```python
from build123d import *

# Parameters (mm, degrees)
F1_DEPTH = 10
F2_W     = 20
F2_H     = 20
F3_DEPTH = 20
F4_SIZE  = 5


with BuildPart() as f1:
    # F0 (on Top) → F1 (new body)
    with BuildSketch(Plane.XY):
        Polygon((0, 20), (0, 0), (40, -20), (40, 20), align=None)
    extrude(amount=F1_DEPTH)

    # F2 (on face) → F3 (join)
    with BuildSketch(Plane.XY.offset(10)):
        with Locations((10, 10)):
            Rectangle(F2_W, F2_H)
    extrude(amount=F3_DEPTH)

    # F4
    f4_edges = [f1.edges().sort_by_distance(p)[0] for p in [
        (0, 10, 30),
        (10, 0, 30),
        (20, 10, 30),
        (10, 20, 30),
    ]]
    chamfer(f4_edges, length=F4_SIZE)


solid = f1.part
```
CAD build for the part. Positions are in the model's coordinates, mm. A direction names the side the tool comes from. Coordinates: 2 decimals unless noted, no trailing zeros. Loops run counter-clockwise (first coordinate to the right, second up) from the corner with the lowest first, then second, coordinate; pieces in that order, holes last. Notation, with made-up numbers: (48, 3.5) - (98, 3.5) arc R19 ccw to (98, 37.5) - close; hole circle Ø7 at (35.5, -19.5). An arc over 180 degrees is marked (long way). Use CSV: the item, a comma, the result in double quotes. Start each with the question number.
Q1. Cut at C-C, the plane z = 6.25. List the corners of the cut face in (x, y), then the cut area to 3 significant figures.
Q2. Cut at B-B, the plane y = 7. List the corners of the cut face in (x, z), then the cut area to 3 significant figures.
Q3. 3-axis set-ups, long thin cutter, end or side, ignore diameter. For faces 1 (the flat face through (20, 10, 17)), 2 (the flat face through (10, 18, 27)), 3 (the flat face through (10, 0, 17)): which of +Z, -Z, +X, -X, +Y, -Y reach the whole face in a straight line?
Q4. Cut at D-D, the plane y = -7. List the corners of the cut face in (x, z), then the cut area to 3 significant figures.
Q5. Probe probe 1 along Z at (x, y) = (16.5, -2); probe 2 along Y at (x, z) = (17, 24). List the from-to ranges inside material, lowest first. Write a range as from..to.
Q6. Drop flat-ended pins along their axis: P1, Ø3, axis at x = 32, y = 3.5, coming from the +Z side; P2, Ø3, axis at x = 32.5, z = 12, coming from the -Y side; P3, Ø1.5, axis at x = 14, z = 27, coming from the +Y side; P4, Ø12, axis at x = 6.5, z = 21, coming from the -Y side. Give the stop position or say it passes through.
Q7. Cut at A-A, the plane x = 12. List the corners of the cut face in (y, z).
Here are the results:
1,outline,"(0, 0) - (40, -20) - (40, 20) - (0, 20) - close"
1,area,"1,200 mm2"
2,outline,"(0, 0) - (40, 0) - (40, 10) - (20, 10) - (20, 25) - (15, 30) - (5, 30) - (0, 25) - close"
2,area,"775 mm2"
3,face 1,"+Z, +X, +Y, -Y"
3,face 2,"+Z, +X, -X, +Y"
3,face 3,"+Z, +X, -X, -Y"
4,outline,"(14, 0) - (40, 0) - (40, 10) - (14, 10) - close"
4,area,"260 mm2"
5,probe 1,"0..10"
5,probe 2,"0..20"
6,P1,"z = 10"
6,P2,"through"
6,P3,"y = 18.75"
6,P4,"y = 0"
7,outline,"(-6, 0) - (20, 0) - (20, 25) - (15, 30) - (5, 30) - (0, 25) - (0, 10) - (-6, 10) - close"
